```python
from build123d import *

# Parameters (mm, degrees)
CROQUIS1_R              = 1.5
SALIENTE_EXTRUIR1_DEPTH = 20
CORTAR_EXTRUIR1_START   = -5
CORTAR_EXTRUIR1_DEPTH   = 5
CORTAR_EXTRUIR2_DEPTH   = 5
CORTAR_EXTRUIR3_DEPTH   = 65.031242374
CROQUIS5_R              = 2
CORTAR_EXTRUIR4_DEPTH   = 10


with BuildPart() as part:
    # Croquis1 → Saliente-Extruir1 (new body)
    # profile 1 of 2: a face of its own
    with BuildSketch(Plane.XY):
        with BuildLine():
            ThreePointArc((7.420644355, 1.088134807), (7.207357835, 25.623325873), (10, 50))
            Line((10, 50), (10, 60))
            Line((10, 60), (-10, 60))
            Line((-10, 60), (-10, 50))
            ThreePointArc((-10, 50), (-7.207357835, 25.623325873), (-7.420644355, 1.088134807))
            ThreePointArc((-7.420644355, 1.088134807), (0, 7.5), (7.420644355, 1.088134807))
        make_face()
    # profile 2 of 2: a face of its own
    with BuildSketch(Plane.XY):
        with BuildLine():
            ThreePointArc((7.5, 0), (7.459580187, 0.544013292), (7.420644355, 1.088134807))
            ThreePointArc((7.420644355, 1.088134807), (0, 7.5), (-7.420644355, 1.088134807))
            ThreePointArc((-7.420644355, 1.088134807), (-7.459580187, 0.544013292), (-7.5, 0))
            ThreePointArc((-7.5, 0), (0, -7.5), (7.5, 0))
        make_face()
        Circle(CROQUIS1_R, mode=Mode.SUBTRACT)
    extrude(amount=SALIENTE_EXTRUIR1_DEPTH)

    # Croquis2 → Cortar-Extruir1 (cut)
    with BuildSketch(Plane.XY.offset(20).offset(CORTAR_EXTRUIR1_START)):
        with BuildLine():
            Line((-7.069523462, 7.617489658), (-6, 7))
            Line((-6, 7), (-2, 7))
            Line((-2, 7), (6.951202379, 12.167979103))
            ThreePointArc((6.951202379, 12.167979103), (7.132948314, 6.079810741), (7.5, 0))
            ThreePointArc((7.5, 0), (0, -7.5), (-7.5, 0))
            ThreePointArc((-7.5, 0), (-7.24843422, 3.806691903), (-7.069523462, 7.617489658))
        make_face()
    extrude(amount=CORTAR_EXTRUIR1_DEPTH, mode=Mode.SUBTRACT)

    # Croquis3 → Cortar-Extruir2 (cut)
    with BuildSketch(Plane(origin=(0, 0, 0), x_dir=(-1, 0, 0), z_dir=(0, 0, -1))):
        with BuildLine():
            Line((-6.951202379, 12.167979103), (2, 7))
            Line((2, 7), (6, 7))
            Line((6, 7), (7.069523462, 7.617489658))
            ThreePointArc((7.069523462, 7.617489658), (7.24843422, 3.806691903), (7.5, 0))
            ThreePointArc((7.5, 0), (0, -7.5), (-7.5, 0))
            ThreePointArc((-7.5, 0), (-7.132948314, 6.079810741), (-6.951202379, 12.167979103))
        make_face()
    extrude(amount=-CORTAR_EXTRUIR2_DEPTH, mode=Mode.SUBTRACT)

    # Croquis4 → Cortar-Extruir3 (cut, through all)
    with BuildSketch(Plane.XY.offset(20)):
        with BuildLine():
            Line((-1.434704258, 13.67722661), (1.429981311, 15.331153594))
            ThreePointArc((1.429981311, 15.331153594), (2.209232224, 32.971789387), (4.5, 50.480405727))
            Line((4.5, 50.480405727), (4.5, 54.5))
            Line((4.5, 54.5), (-4.5, 54.5))
            Line((-4.5, 54.5), (-4.5, 50.480405727))
            ThreePointArc((-4.5, 50.480405727), (-2.13893455, 32.147814145), (-1.434704258, 13.67722661))
        make_face()
    extrude(amount=-CORTAR_EXTRUIR3_DEPTH, mode=Mode.SUBTRACT)

    # Croquis5 → Cortar-Extruir4 (cut)
    with BuildSketch(Plane(origin=(0, 60, 0), x_dir=(1, 0, 0), z_dir=(0, 1, 0))):
        with Locations(Location((0, -10, 0), (0, 0, 270))):
            Circle(CROQUIS5_R)
    extrude(amount=-CORTAR_EXTRUIR4_DEPTH, mode=Mode.SUBTRACT)


solid = part.part
```
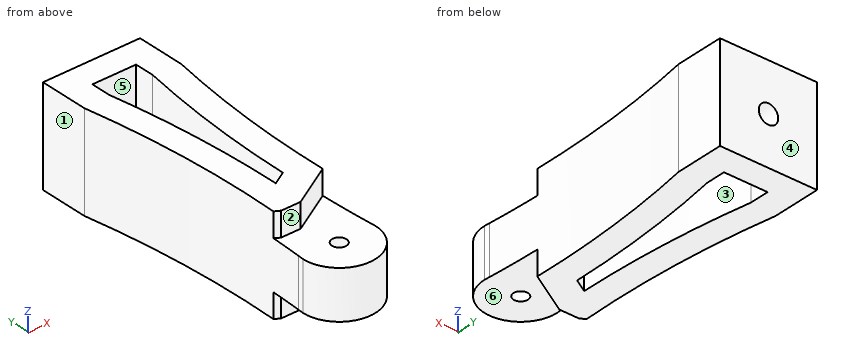
Model file for the job. Use its own axes, mm. Face numbers are marked on the shaded views. A direction names the side the tool comes from. Round coordinates to 2 decimals unless told otherwise and drop trailing zeros. Loops run counter-clockwise (first coordinate to the right, second up) from the corner with the lowest first, then second, coordinate; pieces in that order, holes last. Notation, with made-up numbers: M 10.25,-10.75 L 67.25,-10.75 A12 ccw 67.25,2.25 Z; hole C 55,46.25 d8. An arc over 180 degrees is marked long. Put each result on its own line as item: value. Start each with the question number.
Item 1: Drill centre lines: line 1 along X through (y, z) = (0, 10.25); line 2 along X through (y, z) = (57.05, 10); line 3 along Y through (x, z) = (0, 11.25). Where is each one in solid material? Low to high.
Item 2: 3-axis set-ups, long thin cutter, end or side, ignore diameter. For the marked faces 1, 2 and 3: which of +Z, -Z, +X, -X, +Y, -Y reach the whole face in a straight line?
Item 3: Mould opens along Y. For the marked faces 4, 5 and 6 say: released by +Y, released by -Y, zero draft, split by the parting line, or undercut.
Item 4: Cut at B-B (z = 13.25). List the corners of the cut face in (x, y), then the cut area to 3 significant figures.
Item 5: Cut at C-C (z = 16.5). List the corners of the cut face in (x, y).
Item 6: Cut at D-D (x = 0). List the corners of the cut face in (y, z), then the cut area to 3 significant figures.
Item 7: Cut at A-A (y = 52). List the corners of the cut face in (x, z), then the cut area to 3 significant figures.
Item 8: Drop flat-ended pins along their axis: P1, Ø3, axis at x = -3, z = 17.5, coming from the -Y side; P2, Ø3.5, axis at x = 0, y = 0, coming from the -Z side; P3, Ø3, axis at y = 10, z = 2, coming from the -X side. Give the stop position or say it passes through.
Answer block:
1. line 1: -7.5 to -1.5, 1.5 to 7.5
1. line 2: -10 to -2, 2 to 10
1. line 3: -7.5 to -1.5, 1.5 to 14.51
2. face 1: +Z, -Z, -X, +Y, -Y
2. face 2: +Z, +X, -X, -Y
2. face 3: +Z, -Z
3. face 4: released by +Y
3. face 5: undercut
3. face 6: zero draft
4. outline: M -10,50 A200 cw -7.42,1.09 A200 cw -7.5,0 A7.5 ccw 7.5,0 A200 cw 7.42,1.09 A200 cw 10,50 L 10,60 L -10,60 Z; hole M -4.5,50.48 A205.5 cw -1.43,13.68 L 1.43,15.33 A205.5 cw 4.5,50.48 L 4.5,54.5 L -4.5,54.5 Z; hole C 0,0 d3
4. area: 840 mm2
5. outline: M -10,50 A200 cw -7.07,7.62 L -6,7 L -2,7 L 6.95,12.17 A200 cw 10,50 L 10,60 L -10,60 Z; hole M -4.5,50.48 A205.5 cw -1.43,13.68 L 1.43,15.33 A205.5 cw 4.5,50.48 L 4.5,54.5 L -4.5,54.5 Z
6. outline: M -7.5,5 L -1.5,5 L -1.5,15 L -7.5,15 Z; M 1.5,5 L 8.15,5 L 8.15,0 L 14.51,0 L 14.51,20 L 8.15,20 L 8.15,15 L 1.5,15 Z; M 54.5,0 L 60,0 L 60,8 L 54.5,8 Z; M 54.5,12 L 60,12 L 60,20 L 54.5,20 Z
6. area: 342 mm2
7. outline: M -10,0 L -4.5,0 L -4.5,20 L -10,20 Z; M 4.5,0 L 10,0 L 10,20 L 4.5,20 Z
7. area: 220 mm2
8. P1: y = 7
8. P2: z = 5
8. P3: x = -7.04
